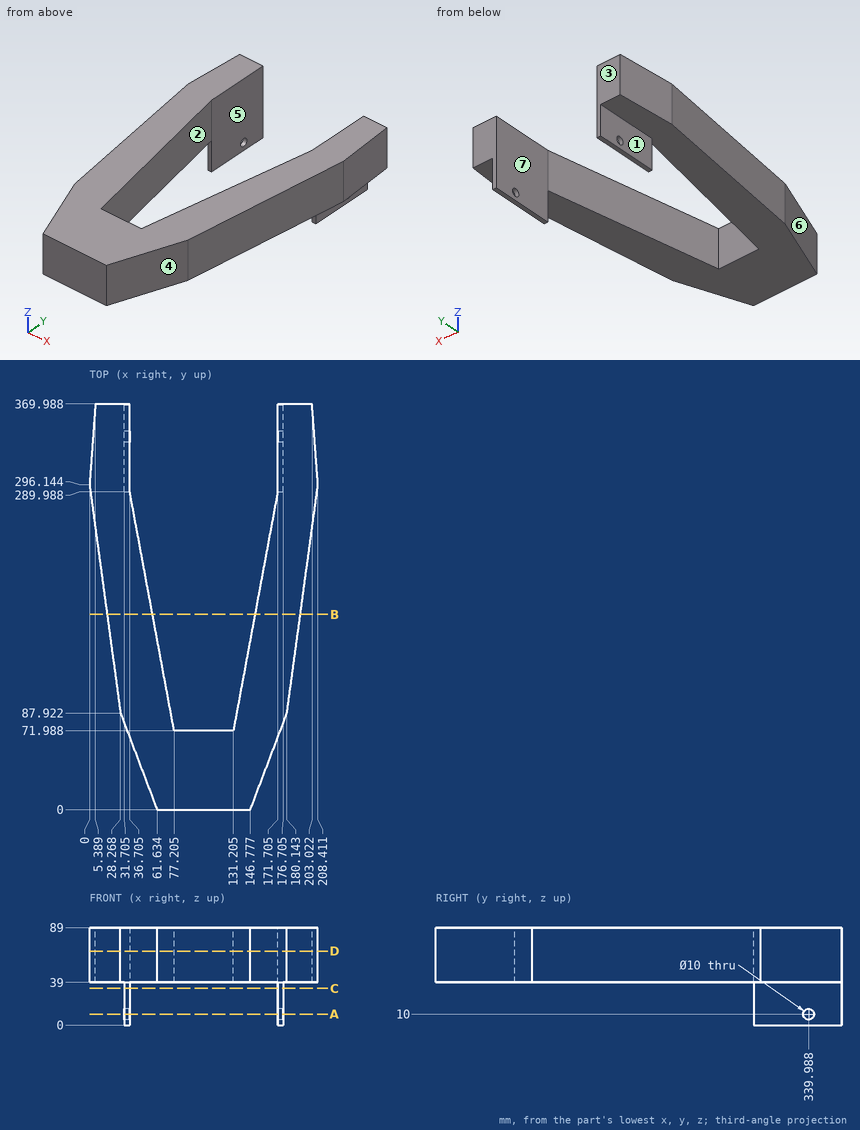
For this review, use the dimensioned drawing (mm, ordinates from the lowest corner) and the shaded views. A direction names the side the tool comes from. Round coordinates to 2 decimals unless told otherwise and drop trailing zeros. Write each loop counter-clockwise with the first axis right and the second up, starting at its lowest first coordinate (ties: lowest second). Pieces come first, ordered by that corner, then holes. Notation, with made-up numbers: M -9,-24.5 L 49,-24.5 A22 ccw 49,12.5 Z; hole C 27.25,33 d2. An arc over 180 degrees is marked long. Use CSV: the item, a comma, the result in double quotes. Start each with the question number.
(1) For line 1 along X through (y, z) = (186, 72) (1 decimal); line 2 along Z through (x, y) = (161, 69.5); line 3 along X through (y, z) = (84.5, 64.5) (1 decimal), list the stretches that pass through material, from the lowest coordinate up.
(2) The part is to be moulded in two halves that separate along X. For the marked faces 4, 5, 6 and 7, say which applies: +X half, -X half, draft (parallel to the pull), parting line (faces both ways), or undercut.
(3) We need section D-D, the plane z = 67.5. State the section outline as (x, y) points (1 decimal), then the cut area to 3 significant figures.
(4) We need section A-A, the plane z = 10. State the section outline as (x, y) points (1 decimal), then the cut area to 3 significant figures.
(5) We need section C-C, the plane z = 33.5. State the section outline as (x, y) points (1 decimal).
(6) Clearance check with flat-ended pins moving along their axes: P1, Ø5.5, axis at x = 174, z = 27.5, coming from the -Y side; P2, Ø5, axis at x = 179, y = 104.5, coming from the -Z side; P3, Ø4, axis at y = 253, z = 51, coming from the +X side (1 decimal). State where each tip first meets the part, or that it passes through.
(7) We need section B-B, the plane y = 178. State the section outline as (x, z) points, then the cut area to 3 significant figures.
(8) Tool access review of the marked faces 1, 2 and 3: name each direction out of +Z, -Z, +X, -X, +Y, -Y from which nothing blocks a thin tool from reaching the whole face with its end or side.
Findings:
1,line 1,"15 to 56, 152.4 to 193.5"
1,line 2,"39 to 89"
1,line 3,"29.6 to 74.9, 133.5 to 178.8"
2,face 4,"+X half"
2,face 5,"undercut"
2,face 6,"-X half"
2,face 7,"undercut"
3,outline,"M 0,296.1 L 28.3,87.9 L 61.6,0 L 146.8,0 L 180.1,87.9 L 208.4,296.1 L 203,370 L 171.7,370 L 171.7,290 L 131.2,72 L 77.2,72 L 36.7,290 L 36.7,370 L 5.4,370 Z"
3,area,"31,500 mm^2"
4,outline,"M 31.7,290 L 36.7,290 L 36.7,335 L 31.7,335 Z; M 31.7,345 L 36.7,345 L 36.7,370 L 31.7,370 Z; M 171.7,290 L 176.7,290 L 176.7,335 L 171.7,335 Z; M 171.7,345 L 176.7,345 L 176.7,370 L 171.7,370 Z"
4,area,"700 mm^2"
5,outline,"M 31.7,290 L 36.7,290 L 36.7,370 L 31.7,370 Z; M 171.7,290 L 176.7,290 L 176.7,370 L 171.7,370 Z"
6,P1,"y = 289.99"
6,P2,"z = 39"
6,P3,"x = 202.8"
7,outline,"M 16.04,39 L 57.51,39 L 57.51,89 L 16.04,89 Z; M 150.9,39 L 192.37,39 L 192.37,89 L 150.9,89 Z"
7,area,"4,150 mm^2"
8,face 1,"-Z, -X, +Y, -Y"
8,face 2,"+Z, -Z, +Y"
8,face 3,"+Z, -Z, +X, -X, +Y"
